Source: three-view drawing plus pictorial views. Frame: mm from the lowest corner of the part. Give positions to 0.01 mm unless a question says otherwise; leave off trailing zeros. Loops run counter-clockwise (first coordinate to the right, second up) from the corner with the lowest first, then second, coordinate; pieces in that order, holes last. Notation, with made-up numbers: (42.25, -17) - (50.25, -17) arc R19 cw to (50.25, 18) - close; hole circle Ø7 at (20, 39). An arc over 180 degrees is marked (long way). Put each result on its own line as item: value.
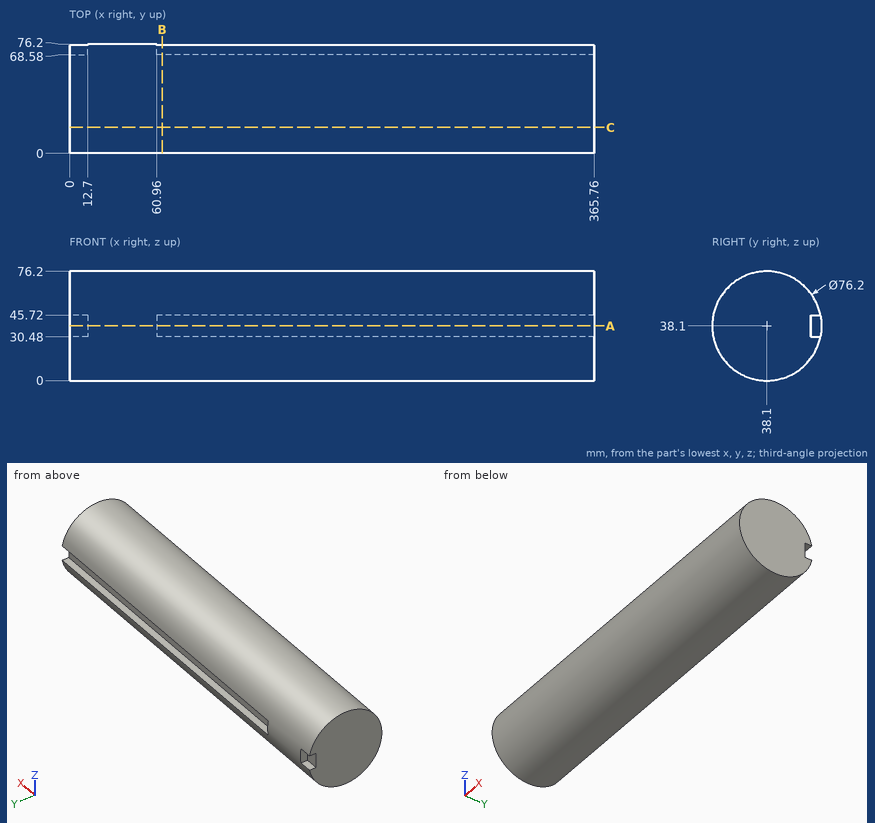
1) Section query A-A, the plane z = 38.1. Output: boundary loops of the cut face in (x, y).
Check result:
outline: (0, 0) - (365.76, 0) - (365.76, 68.58) - (60.96, 68.58) - (60.96, 76.2) - (12.7, 76.2) - (12.7, 68.58) - (0, 68.58) - close
2) Section query B-B, the plane x = 64.5. Output: boundary loops of the cut face in (y, z).
Check result:
outline: (68.58, 30.48) - (68.58, 45.72) - (75.43, 45.72) arc R38.1 ccw (long way) to (75.43, 30.48) - close
3) Pin query (flat end, axial travel): P1, Ø2.5, axis at y = 71, z = 37, coming from the +X side; P2, Ø1.5, axis at x = 311, z = 20, coming from the -Y side; P3, Ø7.5, axis at x = 5.5, y = 73.5, coming from the -Z side. Return the tip coordinate at first contact, or that it passes through.
Check result:
P1: x = 60.96
P2: y = 4.18
P3: z = 16.89
4) Section query C-C, the plane y = 18. Output: boundary loops of the cut face in (x, z), plus the area to 3 significant figures.
Check result:
outline: (0, 5.73) - (365.76, 5.73) - (365.76, 70.47) - (0, 70.47) - close
area: 23,700 mm²
5) Material intervals for line 1 along Z through (x, y) = (183.5, 37.5); line 2 along Y through (x, z) = (341, 40.5); line 3 along Y through (x, z) = (332, 65), sorted ascending. Write a range as [from, to].
Check result:
line 1: [0, 76.2]
line 2: [0.08, 68.58]
line 3: [11.12, 65.08]
